Check sheet for the modelled part. Datum: model origin and axes. Units: mm. Face numbers are marked on the shaded views. Give positions to 0.01 mm unless a question says otherwise; leave off trailing zeros. Loops run counter-clockwise (first coordinate to the right, second up) from the corner with the lowest first, then second, coordinate; pieces in that order, holes last.
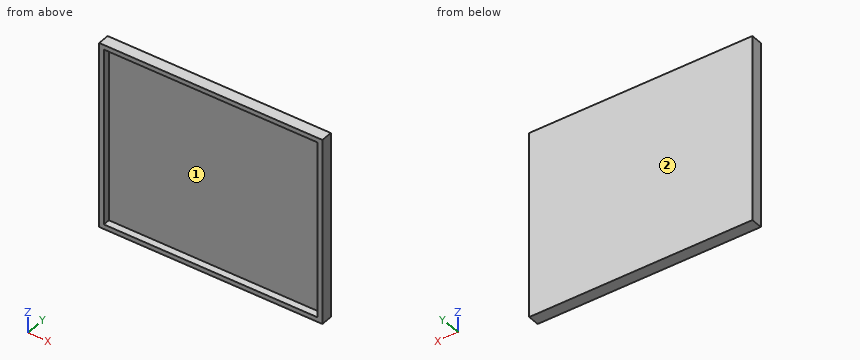
```python
from build123d import *

# Parameters (mm, degrees)
F2_W     = 122.2148686647
F2_H     = 102.0086817443
F3_DEPTH = 6.35
F4_T     = -2.54


# Not quite as in the source:
# - the program builds the solid bodies; features that only make, move or delete a surface that nothing else refers to are left out


with BuildPart() as f3:
    # F2 (on Front) → F3 (new body)
    with BuildSketch(Plane.XZ):
        with Locations((-2.6072487235, 2.9331613332)):
            Rectangle(F2_W, F2_H)
    extrude(amount=F3_DEPTH)

    # F4
    f4_openings = [f3.faces().sort_by_distance(p)[0] for p in [
        (-2.607249, -6.35, 2.933161),
    ]]
    offset(amount=F4_T, openings=f4_openings)


solid = f3.part
```
(1) Release check for a two-part mould opening along X. For the marked faces 1 and 2 record: pulls with the +X half, pulls with the -X half, needs draft (parallel to the pull), parting line crosses it, or undercut.
(2) Material ranges on line 1 (Z direction, x = -54.5, y = -4.25); line 2 (X direction, y = -5, z = 0.5); line 3 (Y direction, x = -2, z = 24), recorded low to high.
(3) Section check B-B on x = -54.5. Record the boundary of the cut face in (y, z), plus the area to 3 significant figures.
(4) Gauge pin test, flat end, axial feed: pin 1 Ø8 at (x, z) = (-49.5, 35.5) entering from -Y. Record the tip position at first contact, or that the pin passes through.
(5) Section check A-A on z = 9. Record the boundary of the cut face in (x, y), plus the area to 3 significant figures.
Computed values:
1. face 1: undercut
1. face 2: needs draft
2. line 1: z = -48.07 to -45.53, 51.4 to 53.94
2. line 2: x = -63.71 to -61.17, 55.96 to 58.5
2. line 3: y = -2.54 to 0
3. outline: (-6.35, -48.07) - (0, -48.07) - (0, 53.94) - (-6.35, 53.94) - (-6.35, 51.4) - (-2.54, 51.4) - (-2.54, -45.53) - (-6.35, -45.53) - close
3. area: 278 mm2
4. pin 1: stops at y = -2.54
5. outline: (-63.71, -6.35) - (-61.17, -6.35) - (-61.17, -2.54) - (55.96, -2.54) - (55.96, -6.35) - (58.5, -6.35) - (58.5, 0) - (-63.71, 0) - close
5. area: 330 mm2
